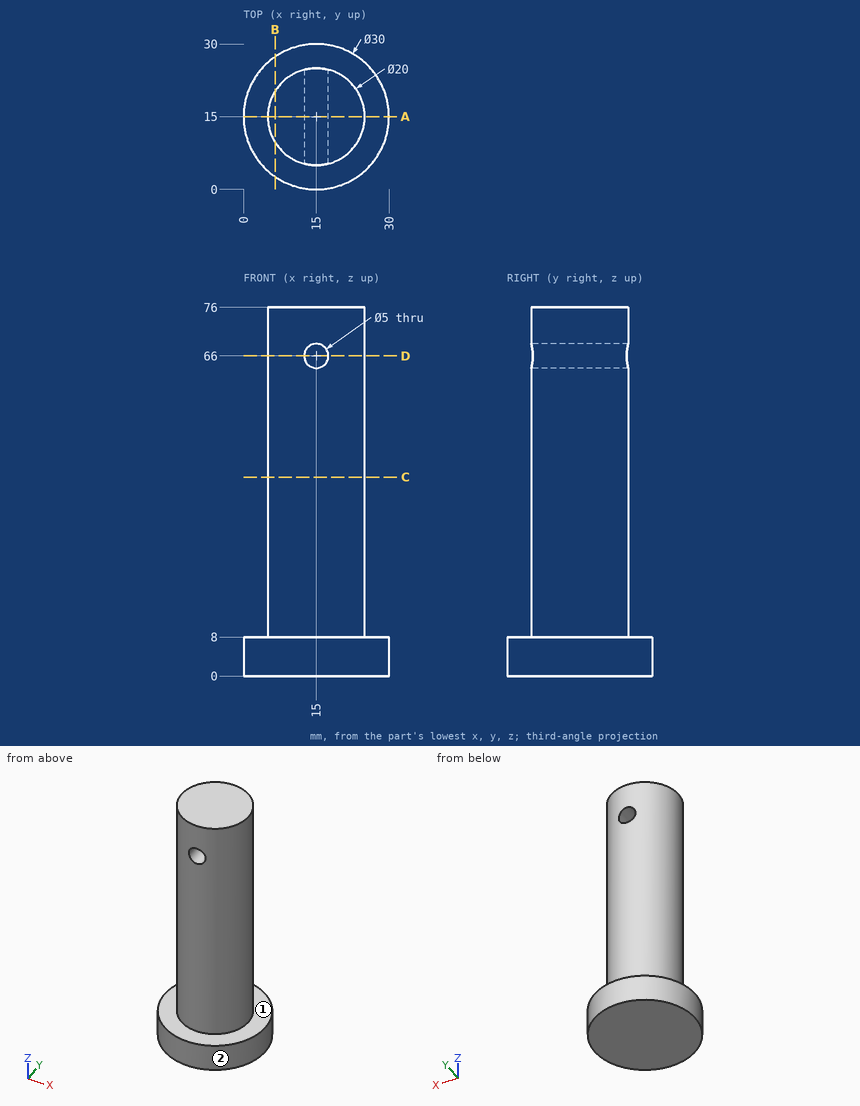
Input: dimensioned drawing with shaded views. Units: mm. Origin: part minimum x, y, z. A direction names the side the tool comes from. Coordinates: 2 decimals unless noted, no trailing zeros. Write each loop counter-clockwise with the first axis right and the second up, starting at its lowest first coordinate (ties: lowest second). Pieces come first, ordered by that corner, then holes. Notation, with made-up numbers: M 19.5,39.25 L 30.5,39.25 A17 ccw 30.5,64.25 Z; hole C 33,-15.75 d10. An arc over 180 degrees is marked long. Answer as CSV lines item,"result". Start each with the question number.
Q1. Cut plane A-A on y = 15. Return the cut outline in (x, z), then the cut area to 3 significant figures.
Q2. Cut plane C-C on z = 41. Return the cut outline in (x, y), then the cut area to 3 significant figures.
Q3. Cut plane B-B on x = 6.5. Return the cut outline in (y, z), then the cut area to 3 significant figures.
Q4. Pin query (flat end, axial travel): P1, Ø8, axis at x = 18.5, y = 8, coming from the -Z side; P2, Ø5, axis at x = 21, z = 22.5, coming from the +Y side; P3, Ø5, axis at y = 3.5, z = 54, coming from the +X side; P4, Ø1.5, axis at y = 17.5, z = 32.5, coming from the +X side. Return the tip coordinate at first contact, or that it passes through.
Q5. Cut plane D-D on z = 66. Return the cut outline in (x, y), then the cut area to 3 significant figures.
Q6. Reachability of the marked faces 1 and 2 from +Z, -Z, +X, -X, +Y, -Y: full face, straight path, thin tool, end or side. Return the list, or none.
Q7. Line query: line 1 (Z direction, x = 15, y = 17.25); line 2 (Z direction, x = 26.5, y = 15.25); line 3 (X direction, y = 14.5, z = 41.5). Output: solid intervals per line, ascending. Write a range as from..to.
Findings below:
1,outline,"M 0,0 L 30,0 L 30,8 L 25,8 L 25,76 L 5,76 L 5,8 L 0,8 Z; hole C 15,66 d5"
1,area,"1,580 mm2"
2,outline,"C 15,15 d20"
2,area,"314 mm2"
3,outline,"M 2.64,0 L 27.36,0 L 27.36,8 L 20.27,8 L 20.27,76 L 9.73,76 L 9.73,8 L 2.64,8 Z"
3,area,"914 mm2"
4,P1,"stops at z = 0"
4,P2,"stops at y = 24.37"
4,P3,"stops at x = 19.36"
4,P4,"stops at x = 24.85"
5,outline,"M 12.5,5.32 L 12.5,24.68 A10 ccw Z; M 17.5,5.32 A10 ccw 17.5,24.68 Z"
5,area,"215 mm2"
6,face 1,"+Z"
6,face 2,"+Z, -Z"
7,line 1,"z = 0..63.5, 68.5..76"
7,line 2,"z = 0..8"
7,line 3,"x = 5.01..24.99"
